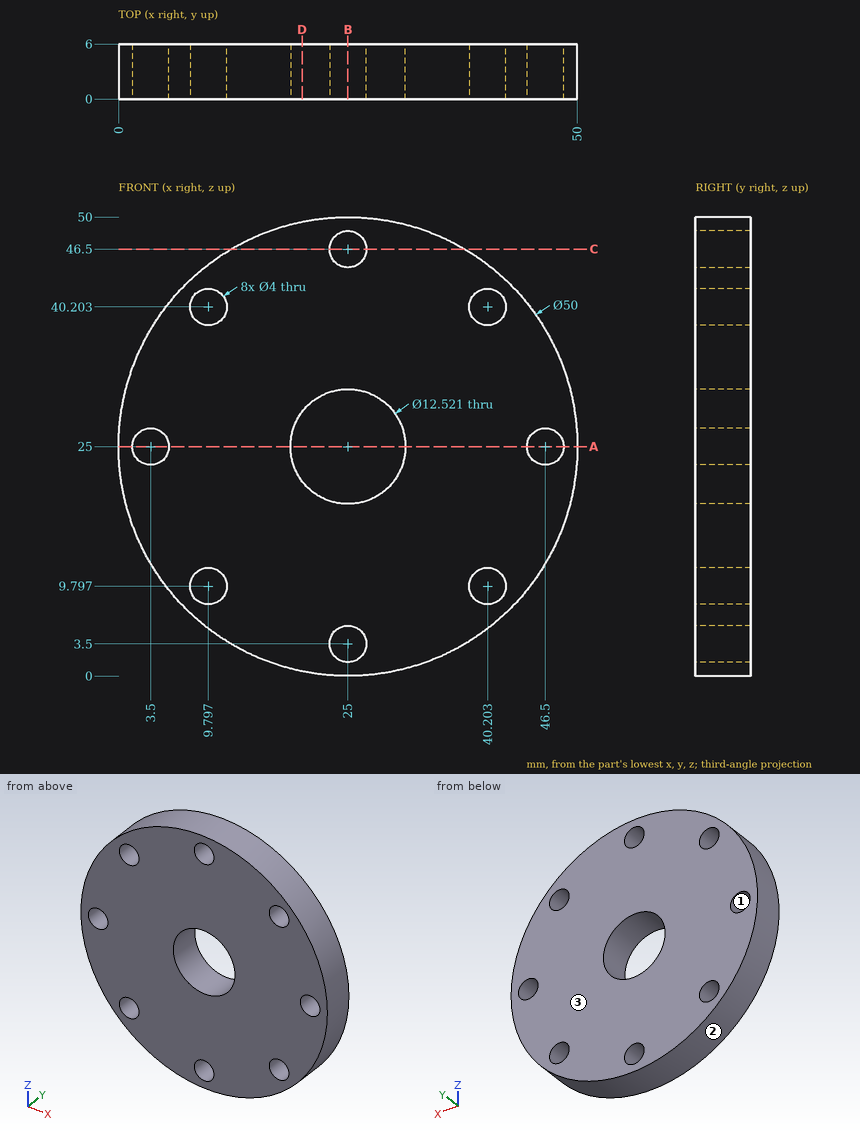
Here's the drawing with two shaded views (mm, measured from the low corner). I have some questions. Give positions to 0.01 mm unless a question says otherwise; leave off trailing zeros. Write each loop counter-clockwise with the first axis right and the second up, starting at its lowest first coordinate (ties: lowest second). Pieces come first, ordered by that corner, then holes. Notation, with made-up numbers: (38.25, -5) -> (96.25, -5) arc R22 ccw to (96.25, 28) -> close; hole circle Ø7 at (-9.5, 38.5). An arc over 180 degrees is marked (long way). Use one line per item in the form item = value. Start each with the question number.
1. Will these pins go through, and if not, where does the flat tip stop? pin 1 Ø2 at (x, y) = (16.5, 1.5) entering from -Z; pin 2 Ø2 at (y, z) = (1, 41.5) entering from -X (1 decimal); pin 3 Ø3.5 at (x, z) = (25, 46.5) entering from +Y; pin 4 Ø1 at (x, y) = (25, 4.5) entering from +Z.
2. Imagine slicing it at C-C on z = 46.5. List the corners of the cut face in (x, y) for me, plus the area to 3 significant figures.
3. Imagine slicing it at D-D on x = 20. List the corners of the cut face in (y, z) for me (1 decimal), plus the area to 3 significant figures.
4. Thinking about a two-plate mould opening in Z: for the marked faces 1, 2 and 3, which applies, +Z half, -Z half, draft (parallel to the pull), parting line (faces both ways), or undercut?
5. Imagine slicing it at A-A on z = 25. List the corners of the cut face in (x, y) for me.
6. If I drill on L1, parallel to X at y = 1.85, z = 25; L2, parallel to X at y = 4.8, z = 42 (1 decimal), over which ranges is the centre line in solid material (lowest first)?
7. Imagine slicing it at B-B on x = 25. List the corners of the cut face in (y, z) for me.
Entries:
q1.pin_1 = 1.15
q1.pin_2 = 5.4
q1.pin_3 = through
q1.pin_4 = 50
q2.outline = (12.24, 0) -> (23, 0) -> (23, 6) -> (12.24, 6) -> close; (27, 0) -> (37.76, 0) -> (37.76, 6) -> (27, 6) -> close
q2.area = 129 mm²
q3.outline = (0, 0.5) -> (6, 0.5) -> (6, 21.2) -> (0, 21.2) -> close; (0, 28.8) -> (6, 28.8) -> (6, 49.5) -> (0, 49.5) -> close
q3.area = 249 mm²
q4.face_1 = undercut
q4.face_2 = parting line
q4.face_3 = draft
q5.outline = (0, 0) -> (1.5, 0) -> (1.5, 6) -> (0, 6) -> close; (5.5, 0) -> (18.74, 0) -> (18.74, 6) -> (5.5, 6) -> close; (31.26, 0) -> (44.5, 0) -> (44.5, 6) -> (31.26, 6) -> close; (48.5, 0) -> (50, 0) -> (50, 6) -> (48.5, 6) -> close
q6.L1 = 0 to 1.5, 5.5 to 18.74, 31.26 to 44.5, 48.5 to 50
q6.L2 = 6.7 to 8.9, 10.7 to 39.3, 41.1 to 43.3
q7.outline = (0, 0) -> (6, 0) -> (6, 1.5) -> (0, 1.5) -> close; (0, 5.5) -> (6, 5.5) -> (6, 18.74) -> (0, 18.74) -> close; (0, 31.26) -> (6, 31.26) -> (6, 44.5) -> (0, 44.5) -> close; (0, 48.5) -> (6, 48.5) -> (6, 50) -> (0, 50) -> close
